The listing builds one solid part. Answer for the finished solid, in the listing's coordinates (mm). Give positions to 0.01 mm unless a question says otherwise; leave off trailing zeros. Write each loop counter-clockwise with the first axis right and the second up, starting at its lowest first coordinate (ties: lowest second). Pieces come first, ordered by that corner, then holes. Notation, with made-up numbers: (47.25, 87.5) - (53.25, 87.5) arc R27 ccw to (53.25, 111.5) - close; hole circle Ø2 at (41, 81). An arc over 180 degrees is marked (long way). One line per item, written item: value. Start each with the question number.
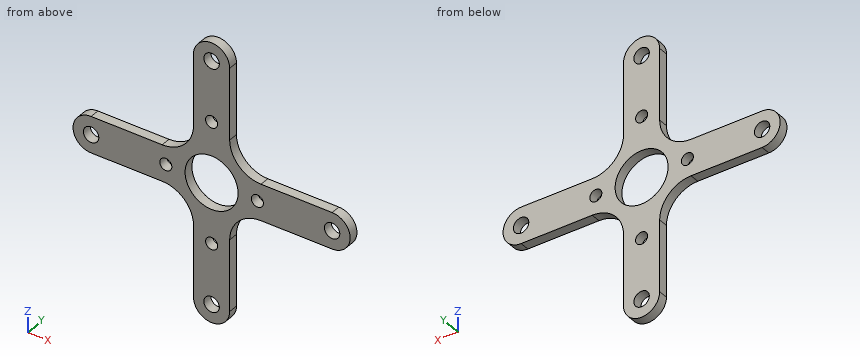
Solid Edge part; units mm, degrees
sketch "Sketch1" plane through (0, 0, 0) normal (0, -1, 0) x (1, 0, 0)
  line L0 (-3.75, 18.75) -> (-3.75, 25)
  arc A0 (-3.75, 25) -> (3.75, 25) centre (0, 25) cw
  line L1 (3.75, 18.75) -> (3.75, 25)
  line L2 (3.75, 10.25) -> (3.75, 18.75)
  arc A1 (3.75, 10.25) -> (10.25, 3.75) centre (10.25, 10.25) ccw
  line L3 (10.25, 3.75) -> (25, 3.75)
  arc A2 (25, 3.75) -> (25, -3.75) centre (25, 0) cw
  line L4 (10.25, -3.75) -> (25, -3.75)
  arc A3 (10.25, -3.75) -> (3.75, -10.25) centre (10.25, -10.25) ccw
  line L5 (3.75, -10.25) -> (3.75, -25)
  arc A4 (3.75, -25) -> (-3.75, -25) centre (0, -25) cw
  line L6 (-3.75, -10.25) -> (-3.75, -25)
  arc A5 (-10.25, -3.75) -> (-3.75, -10.25) centre (-10.25, -10.25) cw
  line L7 (-10.25, -3.75) -> (-25, -3.75)
  arc A6 (-25, -3.75) -> (-25, 3.75) centre (-25, 0) cw
  line L8 (-10.25, 3.75) -> (-25, 3.75)
  arc A7 (-10.25, 3.75) -> (-3.75, 10.25) centre (-10.25, 10.25) ccw
  line L9 (-3.75, 10.25) -> (-3.75, 18.75)
extrude "Protrusion1" add sketch "Sketch1" along normal up to vertex (2 mm away)
sketch "Sketch2" plane through (0, 0, 0) normal (0, -1, 0) x (1, 0, 0)
  circle A0 centre (0, 25) radius 1.6
  circle A1 centre (9.5, 0) radius 1.25
  circle A2 centre (25, 0) radius 1.6
  circle A3 centre (0, 12.5) radius 1.25
  circle A4 centre (-9.5, 0) radius 1.25
  circle A5 centre (-25, 0) radius 1.6
  circle A6 centre (0, -12.5) radius 1.25
  circle A7 centre (0, -25) radius 1.6
  circle A8 centre (0, 0) radius 5.5
extrude "Cutout1" cut sketch "Sketch2" along normal up to next
properties material "Aluminum, 1060"
Item 1: Find section A-A on y = -1.3. Give the number of separate pieces and of enclosed holes in the cut face, plus the area to 3 significant figures.
Item 2: Find section C-C on x = -9.5. Determine the outline of the cut face in (y, z), plus the area to 3 significant figures.
Item 3: Find section B-B on z = 12.5. Determine the outline of the cut face in (x, y).
Item 4: Find section D-D on x = -20.5. Determine the outline of the cut face in (y, z), plus the area to 3 significant figures.
Item 5: Each of these flat-tipped pins is pushed along its axis until it touches: pin 1 Ø14.5 at (x, z) = (0, 0) entering from +Y; pin 2 Ø1 at (y, z) = (-1, 16) entering from +X; pin 3 Ø1 at (y, z) = (-0.5, 16) entering from -X; pin 4 Ø1 at (x, y) = (-17, -1) entering from +Z. Where does it stop, or does it pass through?
Item 6: Straight lines are drawn through the part: line 1 along X through (y, z) = (-0.35, 0); line 2 along Z through (x, y) = (0, -1.1); line 3 along Z through (x, y) = (25, -1.55). For each, find the intervals that lie inside material, in ascending order.
Values:
1. separate pieces: 1
1. enclosed holes: 9
1. area: 672 mm^2
2. outline: (-2, -3.79) - (0, -3.79) - (0, -1.25) - (-2, -1.25) - close; (-2, 1.25) - (0, 1.25) - (0, 3.79) - (-2, 3.79) - close
2. area: 10.2 mm^2
3. outline: (-3.75, -2) - (-1.25, -2) - (-1.25, 0) - (-3.75, 0) - close; (1.25, -2) - (3.75, -2) - (3.75, 0) - (1.25, 0) - close
4. outline: (-2, -3.75) - (0, -3.75) - (0, 3.75) - (-2, 3.75) - close
4. area: 15.0 mm^2
5. pin 1: y = 0
5. pin 2: x = 3.75
5. pin 3: x = -3.75
5. pin 4: z = 3.75
6. line 1: -28.75 to -26.6, -23.4 to -10.75, -8.25 to -5.5, 5.5 to 8.25, 10.75 to 23.4, 26.6 to 28.75
6. line 2: -28.75 to -26.6, -23.4 to -13.75, -11.25 to -5.5, 5.5 to 11.25, 13.75 to 23.4, 26.6 to 28.75
6. line 3: -3.75 to -1.6, 1.6 to 3.75
